Can you work these out from the model? Positions are in its coordinate system, mm. A direction names the side the tool comes from. Give positions to 0.01 mm unless a question says otherwise; leave off trailing zeros. Loops run counter-clockwise (first coordinate to the right, second up) from the corner with the lowest first, then second, coordinate; pieces in that order, holes last.
Solid Edge part; units mm, degrees
sketch "Sketch1" plane through (0, 0, 0) normal (0, 0, 1) x (1, 0, 0)
  circle A0 centre (0, 0) radius 2.725
extrude "Protrusion1" add sketch "Sketch1" against normal blind 3
sketch "Sketch2" plane through (0, 0, 0) normal (0, 0, 1) x (1, 0, 0)
  line L0 (-0.7, -1.2124) -> (-1.05, -0.6062)
  line L1 (-1.4, 0) -> (-1.05, -0.6062)
  line L2 (-1.4, 0) -> (-1.05, 0.6062)
  line L3 (-0.7, 1.2124) -> (-1.05, 0.6062)
  line L4 (-0.7, 1.2124) -> (0, 1.2124)
  line L5 (0.7, 1.2124) -> (0, 1.2124)
  line L6 (0.7, 1.2124) -> (1.05, 0.6062)
  line L7 (1.4, 0) -> (1.05, 0.6062)
  line L8 (1.4, 0) -> (1.05, -0.6062)
  line L9 (0.7, -1.2124) -> (1.05, -0.6062)
  line L10 (0.7, -1.2124) -> (0, -1.2124)
  line L11 (-0.7, -1.2124) -> (0, -1.2124)
extrude "ExtrudedCutout_1" cut sketch "Sketch2" against normal blind 1.45
sketch "Sketch3" plane through (0, 0, -3) normal (0, 0, -1) x (1, 0, 0)
  circle A0 centre (0, 0) radius 1.45
extrude "ExtrudedProtrusion_2" add sketch "Sketch3" along normal blind 25
properties material "Stainless steel"
(1) Please list where these lines run through material, in increasing order: probe 1 along Z at (x, y) = (-0.1, 0.6); probe 2 along Z at (x, y) = (0.7, -1.5); probe 3 along X at (y, z) = (0.1, -6.75).
Returned:
probe 1: z = -28 to -1.45
probe 2: z = -3 to 0
probe 3: x = -1.45 to 1.45
(2) Suppose I cut it at D-D on x = -2.25. List the corners of the cut face in (y, z) for me, plus the area to 3 significant figures.
Returned:
outline: (-1.54, -3) - (1.54, -3) - (1.54, 0) - (-1.54, 0) - close
area: 9.22 mm2
(3) Suppose I cut it at B-B on z = -2.5. List the corners of the cut face in (x, y) for me (3 decimals).
Returned:
outline: circle Ø5.45 at (0, 0)
(4) Which directions (+Z, -Z, +X, -X, +Y, -Y) give clear straight access to the entire face, cutting with the end or side of a thin tool? Please do faces 1 (the flat face through (1.2, -1.2, -3)), 2 (the flat face through (0, 1.212, -1)), 3 (the cylindrical face through (2.6, 0.82, -1.48)).
Returned:
face 1: -Z
face 2: +Z
face 3: +Z, -Z
(5) Suppose I cut it at A-A on x = 0. List the corners of the cut face in (y, z) for me (3 decimals).
Returned:
outline: (-2.725, -3) - (-1.45, -3) - (-1.45, -28) - (1.45, -28) - (1.45, -3) - (2.725, -3) - (2.725, 0) - (1.212, 0) - (1.212, -1.45) - (-1.212, -1.45) - (-1.212, 0) - (-2.725, 0) - close
(6) Suppose I cut it at C-C on z = -17. List the corners of the cut face in (x, y) for me.
Returned:
outline: circle Ø2.9 at (0, 0)
(7) Will these pins go through, and if not, where does the flat tip stop? P1, Ø1.5, axis at y = -0.5, z = -19.5, coming from the +X side; P2, Ø2, axis at y = -0.5, z = -23, coming from the -X side; P3, Ø1.2, axis at x = -0.5, y = 0, coming from the +Z side.
Returned:
P1: stops at x = 1.45
P2: stops at x = -1.45
P3: stops at z = -1.45
(8) Thinking about a two-plate mould opening in Y: for faces 4 (the flat face through (0, 0, -28)), 5 (the cylindrical face through (-1.45, 0.06, -15.32)), 6 (the flat face through (-1.05, 0.61, -0.71)), which applies, pulls with the +Y half, pulls with the -Y half, needs draft (parallel to the pull), parting line crosses it, or undercut?
Returned:
face 4: needs draft
face 5: parting line crosses it
face 6: undercut
